Geometry check sheet. Reference: the model listing, model coordinates, mm. A direction names the side the tool comes from. Round coordinates to 2 decimals unless told otherwise and drop trailing zeros. Loops run counter-clockwise (first coordinate to the right, second up) from the corner with the lowest first, then second, coordinate; pieces in that order, holes last. Notation, with made-up numbers: (-39, 62) - (-16, 62) arc R22 ccw to (-16, 91) - close; hole circle Ø9 at (48.25, 26.25). An arc over 180 degrees is marked (long way). Answer in a Markdown table with one row per item. Add a question column.
```python
from build123d import *

# Parameters (mm, degrees)
SKETCH1_W           = 20
SKETCH1_H           = 40
BOSS_EXTRUDE1_DEPTH = 80
SKETCH8_W           = 16
SKETCH8_H           = 64
BOSS_EXTRUDE2_DEPTH = 57
SKETCH10_R          = 6
CUT_EXTRUDE1_DEPTH  = 51
CUT_EXTRUDE2_DEPTH  = 105.703357948
SKETCH12_W          = 57
SKETCH12_H          = 6
BOSS_EXTRUDE3_DEPTH = 8
SKETCH14_W          = 57
SKETCH14_H          = 6
BOSS_EXTRUDE4_DEPTH = 8
SKETCH17_W          = 48
SKETCH17_H          = 72
CUT_EXTRUDE4_DEPTH  = 36


with BuildPart() as part:
    # Sketch1 → Boss-Extrude1 (new body)
    with BuildSketch(Plane(origin=(0, 0, 0), x_dir=(1, 0, 0), z_dir=(0, 1, 0))):
        Polygon((-17.351649908, 20.312727502), (-57.351649908, -19.687272498), (-17.351649908, -19.687272498), align=None)
        with Locations((-7.351649908, 0.312727502)):
            Rectangle(SKETCH1_W, SKETCH1_H)
    extrude(amount=-BOSS_EXTRUDE1_DEPTH)

    # Sketch8 → Boss-Extrude2 (add)
    with BuildSketch(Plane(origin=(2.648350092, 0, 0), x_dir=(0, 0, -1), z_dir=(1, 0, 0))):
        with Locations((-27.687272498, -40)):
            Rectangle(SKETCH8_W, SKETCH8_H)
    extrude(amount=-BOSS_EXTRUDE2_DEPTH)

    # Sketch10 → Cut-Extrude1 (cut)
    with BuildSketch(Plane(origin=(2.648350092, 0, 0), x_dir=(0, 0, -1), z_dir=(1, 0, 0))):
        with Locations((-27.687272498, -16)):
            Circle(SKETCH10_R)
        with Locations(Location((-27.687272498, -32, 0), (0, 0, 180))):
            Circle(SKETCH10_R)
        with Locations(Location((-27.687272498, -64, 0), (0, 0, 180))):
            Circle(SKETCH10_R)
        with Locations((-27.687272498, -48)):
            Circle(SKETCH10_R)
    extrude(amount=-CUT_EXTRUDE1_DEPTH, mode=Mode.SUBTRACT)

    # Sketch11 → Cut-Extrude2 (cut, through all)
    with BuildSketch(Plane(origin=(0, 0, 0), x_dir=(1, 0, 0), z_dir=(0, 1, 0))):
        Polygon((-47.694795658, -15.687272498), (-15.694795658, 16.312727502), (-5.351649908, 16.312727502), (-5.351649908, -15.687272498), align=None)
    extrude(amount=-CUT_EXTRUDE2_DEPTH, mode=Mode.SUBTRACT)

    # Sketch12 → Boss-Extrude3 (add)
    with BuildSketch(Plane.XZ.offset(72)):
        with Locations((-25.851649908, 32.687272498)):
            Rectangle(SKETCH12_W, SKETCH12_H)
    extrude(amount=BOSS_EXTRUDE3_DEPTH)

    # Sketch14 → Boss-Extrude4 (add)
    with BuildSketch(Plane(origin=(0, -8, 0), x_dir=(1, 0, 0), z_dir=(0, 1, 0))):
        with Locations((-25.851649908, -32.687272498)):
            Rectangle(SKETCH14_W, SKETCH14_H)
    extrude(amount=BOSS_EXTRUDE4_DEPTH)

    # Sketch17 → Cut-Extrude4 (cut)
    with BuildSketch(Plane(origin=(0, 0, -20.312727502), x_dir=(-1, 0, 0), z_dir=(0, 0, -1))):
        with Locations((29.351649908, -40)):
            Rectangle(SKETCH17_W, SKETCH17_H)
    extrude(amount=-CUT_EXTRUDE4_DEPTH, mode=Mode.SUBTRACT)


solid = part.part
```
Q1. Cross-section at B-B, the plane z = -11. Enter the section's corners in (x, y).
Q2. Cross-section at C-C, the plane y = -41. Enter the section's corners in (x, z), plus the area to 3 significant figures.
Q3. Depth check by flat-ended pin: P1, Ø6, axis at y = -15.5, z = 27.5, coming from the +X side; P2, Ø4, axis at x = -51, y = -62.5, coming from the -Z side; P3, Ø1.5, axis at x = -12.5, z = 21.5, coming from the -Y side; P4, Ø4, axis at x = -18, y = -4.5, coming from the -Z side. Enter the tip coordinate at first touch or a pass-through.
Q4. Scan lines: line 1 (Z direction, x = -26, y = -32); line 2 (Z direction, x = -42, y = -40); line 3 (X direction, y = -59, z = 10.5). Record each from-to range of solid material in increasing order. Write a range as from..to.
Q5. Cross-section at D-D, the plane x = -37. Enter the section's corners in (y, z).
Q6. Cross-section at A-A, the plane x = -8.5. Enter the section's corners in (y, z), plus the area to 3 significant figures.
Q7. Release check for a two-part mould opening along X. For faces 5 (the flat face through (-48.352, -32, 28)), 6 (the flat face through (-31.92, -1.97, -0.09)), 7 (the flat face through (-26, -41, 35.687)) record: +X half, -X half, draft (parallel to the pull), parting line (faces both ways), or undercut.
Q8. Set-up check for faces 1 (the cylindrical face through (-22.49, -26.14, 26.39)), 2 (the flat face through (-11, -78, -16.313)), 3 (the flat face through (-29, -76, -5)), 4 (the flat face through (-25, -72, 25)): record each of +Z, -Z, +X, -X, +Y, -Y from which the full face is reachable in a straight line by a thin tool's end or side.
Check sheet entries:
| question | item | result |
|---|---|---|
| 1 | outline | (-26.66, -80) - (-21.01, -80) - (-21.01, -76) - (-26.66, -76) - close; (-26.66, -4) - (-21.01, -4) - (-21.01, 0) - (-26.66, 0) - close; (-5.35, -80) - (2.65, -80) - (2.65, 0) - (-5.35, 0) - close |
| 2 | outline | (-57.35, 19.69) - (-53.35, 15.69) - (-5.35, 15.69) - (-5.35, -20.31) - (2.65, -20.31) - (2.65, 35.69) - (-54.35, 35.69) - (-54.35, 19.69) - close |
| 2 | area | 1,430 mm² |
| 3 | P1 | x = -48.35 |
| 3 | P2 | z = 15.69 |
| 3 | P3 | y = -72 |
| 3 | P4 | z = -20.31 |
| 4 | line 1 | 15.69..21.69, 33.69..35.69 |
| 4 | line 2 | 15.69..35.69 |
| 4 | line 3 | -5.35..2.65 |
| 5 | outline | (-80, -0.66) - (-76, -0.66) - (-76, 4.99) - (-80, 4.99) - close; (-80, 15.69) - (0, 15.69) - (0, 19.69) - (-8, 19.69) - (-8, 29.69) - (0, 29.69) - (0, 35.69) - (-80, 35.69) - (-80, 29.69) - (-72, 29.69) - (-72, 19.69) - (-80, 19.69) - close; (-4, -0.66) - (0, -0.66) - (0, 4.99) - (-4, 4.99) - close; hole circle Ø12 at (-64, 27.69); hole circle Ø12 at (-48, 27.69); hole circle Ø12 at (-32, 27.69); hole circle Ø12 at (-16, 27.69) |
| 6 | outline | (-80, -20.31) - (-76, -20.31) - (-76, -16.31) - (-80, -16.31) - close; (-80, 15.69) - (0, 15.69) - (0, 19.69) - (-8, 19.69) - (-8, 29.69) - (0, 29.69) - (0, 35.69) - (-80, 35.69) - (-80, 29.69) - (-72, 29.69) - (-72, 19.69) - (-80, 19.69) - close; (-4, -20.31) - (0, -20.31) - (0, -16.31) - (-4, -16.31) - close; hole circle Ø12 at (-64, 27.69); hole circle Ø12 at (-48, 27.69); hole circle Ø12 at (-32, 27.69); hole circle Ø12 at (-16, 27.69) |
| 6 | area | 1,020 mm² |
| 7 | face 5 | +X half |
| 7 | face 6 | undercut |
| 7 | face 7 | draft |
| 8 | face 1 | +X |
| 8 | face 2 | +Y, -Y |
| 8 | face 3 | -Z, -X |
| 8 | face 4 | +X, -X, -Y |
